Geometry check sheet. Reference: the model listing, model coordinates, mm. A direction names the side the tool comes from. Give positions to 0.01 mm unless a question says otherwise; leave off trailing zeros. Write each loop counter-clockwise with the first axis right and the second up, starting at its lowest first coordinate (ties: lowest second). Pieces come first, ordered by that corner, then holes. Notation, with made-up numbers: M -22.5,-20.75 L 22.5,-20.75 A11 cw 22.5,-14.75 Z; hole C -31.75,-10 d6. An arc over 180 degrees is marked long. Use one line per item in the form item = value. Start each with the question number.
Autodesk Inventor part; units mm, degrees
ref_plane "YZ Plane" through (0, 0, 0) normal (1, 0, 0) x (0, 1, 0)
ref_plane "XZ Plane" through (0, 0, 0) normal (0, 1, 0) x (-1, 0, 0)
ref_plane "XY Plane" through (0, 0, 0) normal (0, 0, 1) x (1, 0, 0)
sketch "Sketch1" plane through (0, 0, 0) normal (0, 0, 1) x (1, 0, 0)
  circle A0 centre (0, 0) radius 4
  line L0 (-1.555751, 4.751804) -> (1.555751, 4.751804)
  line L1 (0, 0) -> (1.555751, 0)
  line L2 (-1.555751, -4.751804) -> (1.555751, -4.751804)
  arc A1 (-1.555751, 4.751804) -> (-1.555751, -4.751804) centre (0, 0) ccw
  arc A2 (1.555751, -4.751804) -> (1.555751, 4.751804) centre (0, 0) ccw
  circle A3 centre (0, 0) radius 4.5
  dimension "d0" = 8
  dimension "d2" = 9
extrude "Extrusion1" add sketch "Sketch1" along normal blind 27.5 contours A0
extrude "Extrusion2" add sketch "Sketch1" along normal blind 22.5 contours A3
sketch "Sketch2" plane through (0, 0, 22.5) normal (0, 0, 1) x (1, 0, 0)
  circle A0 centre (0, 0) radius 5.629087
  line L0 (0, 0) -> (1.158118, 0)
  line L1 (-1.971905, 5.2724) -> (1.971905, 5.2724)
  line L2 (-1.971905, -5.2724) -> (1.971905, -5.2724)
extrude "Extrusion3" add sketch "Sketch2" against normal blind 5 contours A0 L2 L1
sketch "Sketch3" plane through (0, 0, 0) normal (0, 0, -1) x (-1, 0, 0)
  circle A0 centre (0, 0) radius 4.5
  line L0 (-2.019433, 4.021429) -> (2.019433, 4.021429)
  line L1 (0, 0) -> (1.467716, 0)
  line L2 (-2.019433, -4.021429) -> (2.019433, -4.021429)
  arc A1 (2.019433, 4.021429) -> (-2.019433, 4.021429) centre (0, 0) ccw
  arc A2 (-2.019433, -4.021429) -> (2.019433, -4.021429) centre (0, 0) ccw
extrude "Extrusion4" cut sketch "Sketch3" against normal blind 3 contours L0 A0 | A0 L2
sketch "Sketch4" plane through (0, 0, 0) normal (0, 1, 0) x (-1, 0, 0)
  circle A0 centre (0, -7.5) radius 7.5
  line L0 (2.019433, 0) -> (-2.019433, 0)
  line L1 (-2.019433, 0) -> (-4.5, 0)
  line L2 (-4.5, 0) -> (4.599623, 0)
  arc A1 (-4.5, 0) -> (-6.78711, -4.308583) centre (38.772452, -25.731481) ccw
  line L3 (4.599623, 0) -> (6.684935, -4.099757)
  line L4 (-4.5, 0) -> (4.599623, 0)
  point P0 (0, 0)
  point P1 (0, 0)
  dimension "d11" = 15
  dimension "d12" = 7.5
extrude "Extrusion5" add sketch "Sketch4" against normal blind 1
extrude "Extrusion6" add sketch "Sketch4" along normal blind 1
sketch "Sketch6" plane through (0, 1, 0) normal (0, 1, 0) x (1, 0, 0)
  arc A0 (6.78711, 4.308583) -> (-6.684935, 4.099757) centre (0, 7.5) ccw
  circle A1 centre (0, 7.5) radius 5
  point P0 (0, 0)
  dimension "d17" = 10
extrude "Extrusion7" cut sketch "Sketch6" against normal blind 2
fillet "Fillet1" radius 2 2 edges at (0, 1, 0) (0, -1, 0)
fillet "Fillet2" radius 1 2 edges at (0, -4.0214, 0) (0, 4.0214, 0)
fillet "Fillet3" radius 0.5 6 edges at (-5.6423, 1, -2.0499) (5.6958, 1, -2.1266) (-0.1162, 1, -14.9991) (5.6958, -1, -2.1266) (-5.6423, -1, -2.0499) (-0.1162, -1, -14.9991)
equation "\"BendRadius\" = Thickness"
equation "\"BendReliefWidth\" = Thickness"
equation "\"BendReliefDepth\" = 0.5 * Thickness"
equation "\"CornerReliefSize\" = 4 * Thickness"
equation "\"MinimumRemnant\" = 2 * Thickness"
equation "\"TransitionRadius\" = BendRadius"
equation "\"JacobiRadiusSize\" = BendRadius"
equation "\"GapSize\" = Thickness"
properties part number "vòng bi_dài 35mm"
(1) Thickness scan on probe 1 along Z at (x, y) = (0, 0.55); probe 2 along X at (y, z) = (0.05, -7.5); probe 3 along X at (y, z) = (2, 8). Record the ranges inside material, lowest first. Write a range as [from, to].
(2) Depth check by flat-ended pin: pin 1 (0.6 mm diameter, centred on x = -0.5, z = 2, fed in from -Y); pin 2 (8 mm diameter, centred on x = 0, z = -7.5, fed in from +Y); pin 3 (7 mm diameter, centred on x = -3.5, z = -8, fed in from +Y); pin 4 (6 mm diameter, centred on y = 1.5, z = 16.5, fed in from +X). Enter the tip coordinate at first touch or a pass-through.
(3) Sectioned sample at C-C, the plane y = -1.5. Record the boundary of the cut face in (x, z).
(4) Sectioned sample at B-B, the plane z = -7.5. Record the boundary of the cut face in (x, y), plus the area to 3 significant figures.
(5) Sectioned sample at D-D, the plane z = 16. Record the boundary of the cut face in (x, y), plus the area to 3 significant figures.
(6) Draft check along Z on faces 1 (the cylindrical face through (-0.06, 1.57, -0.6)), 2 (the flat face through (0, 4.021, 2)), 3 (the cylindrical face through (-5.48, -0.85, -2.05)). Enter one of: released by +Z, released by -Z, zero draft, split by the parting line, or undercut.
(7) Tool access check on faces 4 (the flat face through (0, -4.021, 2)), 5 (the flat face through (5, 0, 17.5)), 6 (the flat face through (-5.628, -0.007, -2.021)), 7 (the cylindrical face through (-0.867, 3.905, 24.965)). Record the directions out of +Z, -Z, +X, -X, +Y, -Y that give a thin tool (end or side, any length) a straight path to the whole face; none if there is none.
Numbers:
q1.probe_1 = [-15, -12.5], [-2.5, 27.5]
q1.probe_2 = [-7.5, -5], [5, 7.5]
q1.probe_3 = [-4.03, 4.03]
q2.pin_1 = -4.02
q2.pin_2 = through
q2.pin_3 = 1
q2.pin_4 = 5.63
q3.outline = M -5.43,17.5 L -4.24,17.5 L -4.24,-0.68 L 4.24,-0.68 L 4.24,17.5 L 5.43,17.5 L 5.43,22.5 L 3.71,22.5 L 3.71,27.5 L -3.71,27.5 L -3.71,22.5 L -5.43,22.5 Z
q4.outline = M -7.5,-0.5 A0.5 ccw -7,-1 L -5,-1 L -5,1 L -7,1 A0.5 ccw -7.5,0.5 Z; M 5,-1 L 7,-1 A0.5 ccw 7.5,-0.5 L 7.5,0.5 A0.5 ccw 7,1 L 5,1 Z
q4.area = 9.79 mm2
q5.outline = C 0,0 d9
q5.area = 63.6 mm2
q6.face_1 = released by -Z
q6.face_2 = zero draft
q6.face_3 = undercut
q7.face_4 = -Z, +X, -X, -Y
q7.face_5 = none
q7.face_6 = -X, +Y, -Y
q7.face_7 = +Z
